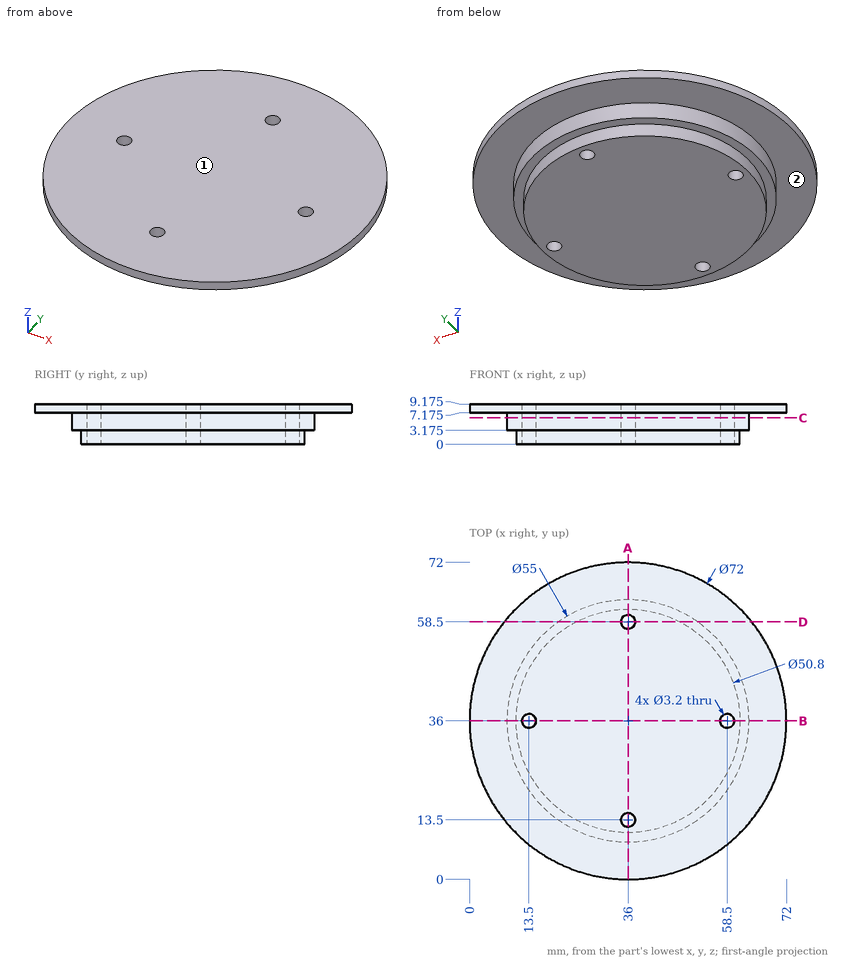
Drawing for the job (mm, zero at the part's lowest x, y, z). A direction names the side the tool comes from. Round coordinates to 2 decimals unless told otherwise and drop trailing zeros. Loops run counter-clockwise (first coordinate to the right, second up) from the corner with the lowest first, then second, coordinate; pieces in that order, holes last. Notation, with made-up numbers: (54.5, 84) -> (70.5, 84) arc R8 cw to (70.5, 92) -> close; hole circle Ø4 at (57.25, 15.25). An arc over 180 degrees is marked (long way). Answer in a Markdown table with one row per item.
Item 1: Saw through at C-C (z = 6). Write the cut outline in (x, y).
Answers below:
| item | result |
|---|---|
| outline | circle Ø55 at (36, 36); hole circle Ø3.2 at (13.5, 36); hole circle Ø3.2 at (36, 13.5); hole circle Ø3.2 at (36, 58.5); hole circle Ø3.2 at (58.5, 36) |
Item 2: Drill centre lines: L1, parallel to Y at x = 36, z = 5.75; L2, parallel to Z at x = 13.5, y = 49 (3 decimals); L3, parallel to Z at x = 4, y = 35.5 (3 decimals). Where is each one in solid material? Low to high. Write a range as [from, to].
Answers below:
| item | result |
|---|---|
| L1 | y = [8.5, 11.9], [15.1, 56.9], [60.1, 63.5] |
| L2 | z = [3.175, 9.175] |
| L3 | z = [7.175, 9.175] |
Item 3: Saw through at A-A (x = 36). Write the cut outline in (y, z) (3 decimals).
Answers below:
| item | result |
|---|---|
| outline | (0, 7.175) -> (8.5, 7.175) -> (8.5, 3.175) -> (10.6, 3.175) -> (10.6, 0) -> (11.9, 0) -> (11.9, 9.175) -> (0, 9.175) -> close; (15.1, 0) -> (56.9, 0) -> (56.9, 9.175) -> (15.1, 9.175) -> close; (60.1, 0) -> (61.4, 0) -> (61.4, 3.175) -> (63.5, 3.175) -> (63.5, 7.175) -> (72, 7.175) -> (72, 9.175) -> (60.1, 9.175) -> close |
Item 4: Pin check, flat tips, straight feed: pin 1 (3 mm diameter, centred on x = 36, y = 58.5, fed in from +Z); pin 2 (1.5 mm diameter, centred on y = 51, z = 8, fed in from +X); pin 3 (3 mm diameter, centred on y = 50.5, z = 7.5, fed in from +X); pin 4 (5 mm diameter, centred on y = 57.5, z = 5, fed in from +X). Stop position of each tip, or through.
Answers below:
| item | result |
|---|---|
| pin 1 | passes through |
| pin 2 | stops at x = 69.06 |
| pin 3 | stops at x = 69.57 |
| pin 4 | stops at x = 65.75 |
Item 5: Saw through at D-D (y = 58.5). Write the cut outline in (x, z) (1 decimal), and give its area (3 significant figures).
Answers below:
| item | result |
|---|---|
| outline | (7.9, 7.2) -> (20.2, 7.2) -> (20.2, 3.2) -> (24.2, 3.2) -> (24.2, 0) -> (34.4, 0) -> (34.4, 9.2) -> (7.9, 9.2) -> close; (37.6, 0) -> (47.8, 0) -> (47.8, 3.2) -> (51.8, 3.2) -> (51.8, 7.2) -> (64.1, 7.2) -> (64.1, 9.2) -> (37.6, 9.2) -> close |
| area | 284 mm² |
Item 6: Which spindle directions (+Z, -Z, +X, -X, +Y, -Y) get a long thin tool onto all of the face, cutting with end or side? Do the marked faces 1 and 2. Say none if no direction does.
Answers below:
| item | result |
|---|---|
| face 1 | +Z, +X, -X, +Y, -Y |
| face 2 | -Z |
